Could you check a few things on this model? Use its own coordinates, in mm. Coordinates: 2 decimals unless noted, no trailing zeros. Loops run counter-clockwise (first coordinate to the right, second up) from the corner with the lowest first, then second, coordinate; pieces in that order, holes last.
from build123d import *

# Parameters (mm, degrees)
SKETCH_R   = 30
SKETCH_R_2 = 3
PAD_DEPTH  = 6


with BuildPart() as part:
    # Sketch → Pad (new body)
    with BuildSketch(Plane.XY):
        Polygon((44, 115), (44, 0), (-44, 0), (-44, 115), (-15.375644, 115), (-13.5, 108), (13.5, 108), (15.375644, 115), align=None)
        with Locations((0, 60)):
            Circle(SKETCH_R, mode=Mode.SUBTRACT)
        with Locations((-34.8, 94.8)):
            Circle(SKETCH_R_2, mode=Mode.SUBTRACT)
        with Locations((34.8, 94.8)):
            Circle(SKETCH_R_2, mode=Mode.SUBTRACT)
        with Locations((-34.8, 25.2)):
            Circle(SKETCH_R_2, mode=Mode.SUBTRACT)
        with Locations((34.8, 25.2)):
            Circle(SKETCH_R_2, mode=Mode.SUBTRACT)
        with BuildLine():
            ThreePointArc((-22, 110), (-25, 113), (-28, 110))
            Line((-28, 110), (-28, 105))
            ThreePointArc((-28, 105), (-25, 102), (-22, 105))
            Line((-22, 110), (-22, 105))
        make_face(mode=Mode.SUBTRACT)
        with BuildLine():
            ThreePointArc((28, 110), (25, 113), (22, 110))
            Line((22, 110), (22, 105))
            ThreePointArc((22, 105), (25, 102), (28, 105))
            Line((28, 110), (28, 105))
        make_face(mode=Mode.SUBTRACT)
        with BuildLine():
            ThreePointArc((28, 10), (25, 13), (22, 10))
            Line((22, 10), (22, 5))
            ThreePointArc((22, 5), (25, 2), (28, 5))
            Line((28, 10), (28, 5))
        make_face(mode=Mode.SUBTRACT)
        with BuildLine():
            ThreePointArc((-22, 10), (-25, 13), (-28, 10))
            Line((-28, 10), (-28, 5))
            ThreePointArc((-28, 5), (-25, 2), (-22, 5))
            Line((-22, 10), (-22, 5))
        make_face(mode=Mode.SUBTRACT)
    extrude(amount=PAD_DEPTH)


solid = part.part
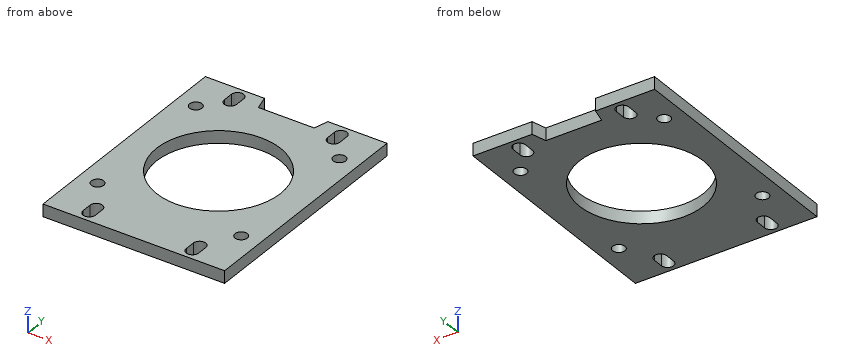
1) Imagine slicing it at B-B on x = -6.5. List the corners of the cut face in (y, z) for me, plus the area to 3 significant figures.
2) Imagine slicing it at A-A on y = 60. List the corners of the cut face in (x, z) for me, plus the area to 3 significant figures.
3) If I drill on L1, parallel to Y at x = -34.8, z = 1.35; L2, parallel to Y at x = 23, z = 1.9; L3, parallel to Y at x = 0, z = 1.3, over which ranges is the centre line in solid material (lowest first)?
4) Will these pins go through, and if not, where does the flat tip stop? pin 1 (5 mm diameter, centred on x = -34.8, y = 94.8, fed in from -Z); pin 2 (3 mm diameter, centred on x = -3.5, z = 2.5, fed in from +Y).
5) Imagine slicing it at C-C on z = 4.35. State how many separate pieces and enclosed holes the cut face has, plus the area to 3 significant figures.
6) Imagine slicing it at D-D on y = 94.8. List the corners of the cut face in (x, z) for me, plus the area to 3 significant figures.
Solved:
1. outline: (0, 0) - (30.71, 0) - (30.71, 6) - (0, 6) - close; (89.29, 0) - (108, 0) - (108, 6) - (89.29, 6) - close
1. area: 297 mm2
2. outline: (-44, 0) - (-30, 0) - (-30, 6) - (-44, 6) - close; (30, 0) - (44, 0) - (44, 6) - (30, 6) - close
2. area: 168 mm2
3. L1: y = 0 to 22.2, 28.2 to 91.8, 97.8 to 115
3. L2: y = 0 to 2.76, 12.24 to 40.74, 79.26 to 102.76, 112.24 to 115
3. L3: y = 0 to 30, 90 to 108
4. pin 1: passes through
4. pin 2: stops at y = 108
5. separate pieces: 1
5. enclosed holes: 9
5. area: 6,740 mm2
6. outline: (-44, 0) - (-37.8, 0) - (-37.8, 6) - (-44, 6) - close; (-31.8, 0) - (31.8, 0) - (31.8, 6) - (-31.8, 6) - close; (37.8, 0) - (44, 0) - (44, 6) - (37.8, 6) - close
6. area: 456 mm2
